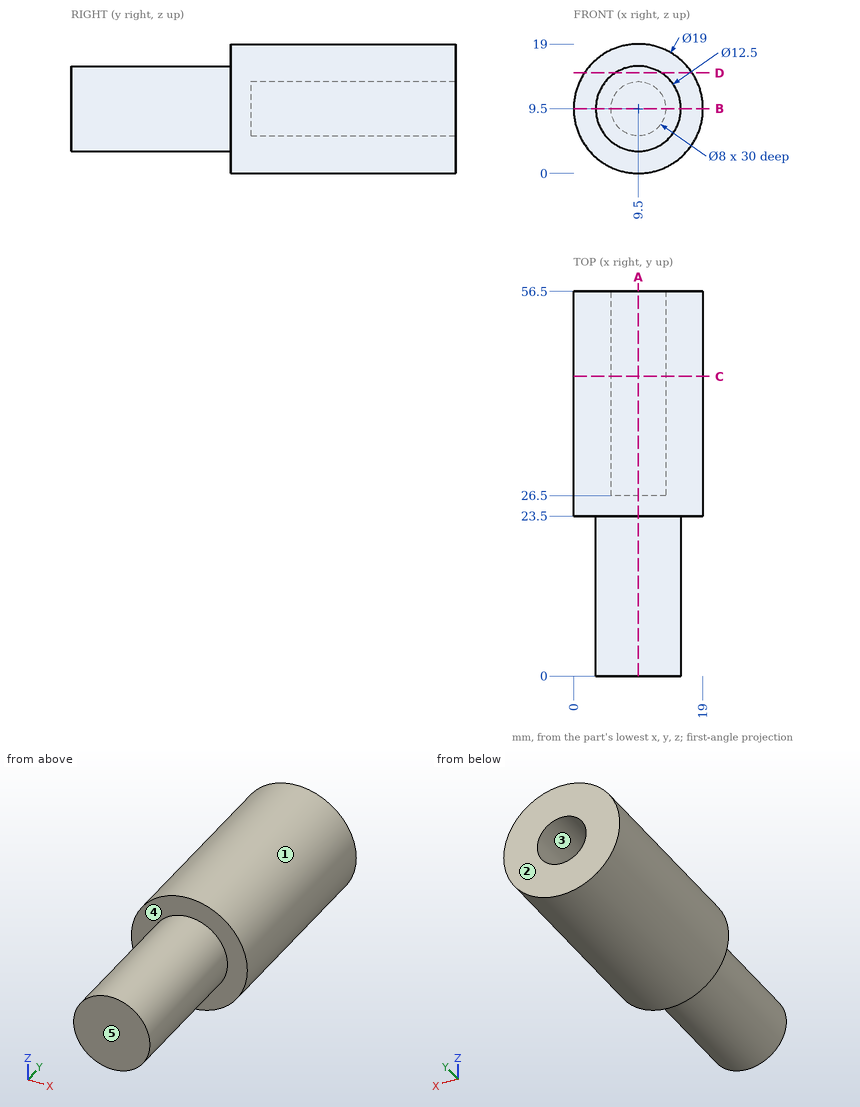
Part print with two shaded views. Sizes in mm from the minimum x, y, z corner. A direction names the side the tool comes from. Coordinates: 2 decimals unless noted, no trailing zeros. Order: outer loops, then holes, each group sorted by start corner. A loop starts at its lowest first (then second) coordinate and runs counter-clockwise, first axis right, second up.
(1) Which spindle directions (+Z, -Z, +X, -X, +Y, -Y) get a long thin tool onto all of the face, cutting with end or side? Do the marked faces 4 and 5. Say none if no direction does.
Solution:
face 4: -Y
face 5: +Z, -Z, +X, -X, -Y
(2) Saw through at A-A, the plane x = 9.5. Write the cut outline in (y, z), and give its area (3 significant figures).
Solution:
outline: (0, 3.25) - (23.5, 3.25) - (23.5, 0) - (56.5, 0) - (56.5, 5.5) - (26.5, 5.5) - (26.5, 13.5) - (56.5, 13.5) - (56.5, 19) - (23.5, 19) - (23.5, 15.75) - (0, 15.75) - close
area: 681 mm2
(3) Saw through at D-D, the plane z = 14.75. Write the cut outline in (x, y).
Solution:
outline: (1.58, 23.5) - (6.11, 23.5) - (6.11, 0) - (12.89, 0) - (12.89, 23.5) - (17.42, 23.5) - (17.42, 56.5) - (1.58, 56.5) - close
(4) Mould opens along Z. For the marked faces 1, 2 and 3 say: released by +Z, released by -Z, zero draft, split by the parting line, or undercut.
Solution:
face 1: split by the parting line
face 2: zero draft
face 3: undercut
(5) Saw through at C-C, the plane y = 44. Write the cut outline in (x, z), and give its area (3 significant figures).
Solution:
outline: circle Ø19 at (9.5, 9.5); hole circle Ø8 at (9.5, 9.5)
area: 233 mm2
(6) Saw through at B-B, the plane z = 9.5. Write the cut outline in (x, y), and give its area (3 significant figures).
Solution:
outline: (0, 23.5) - (3.25, 23.5) - (3.25, 0) - (15.75, 0) - (15.75, 23.5) - (19, 23.5) - (19, 56.5) - (13.5, 56.5) - (13.5, 26.5) - (5.5, 26.5) - (5.5, 56.5) - (0, 56.5) - close
area: 681 mm2
(7) Drill centre lines: L1, parallel to Z at x = 9.25, y = 44; L2, parallel to Y at x = 14.5, z = 17.25; L3, parallel to Z at x = 8, y = 53. Where is each one in solid material? Low to high.
Solution:
L1: z = 0 to 5.51, 13.49 to 19
L2: y = 23.5 to 56.5
L3: z = 0.12 to 5.79, 13.21 to 18.88
(8) Pin check, flat tips, straight feed: pin 1 Ø4 at (x, y) = (5, 17.5) entering from -Z; pin 2 Ø1 at (x, y) = (16.5, 47) entering from -Z; pin 3 Ø1 at (y, z) = (35.5, 3.5) entering from +X. Stop position of each tip, or through.
Solution:
pin 1: stops at z = 3.77
pin 2: stops at z = 2.57
pin 3: stops at x = 17.25
